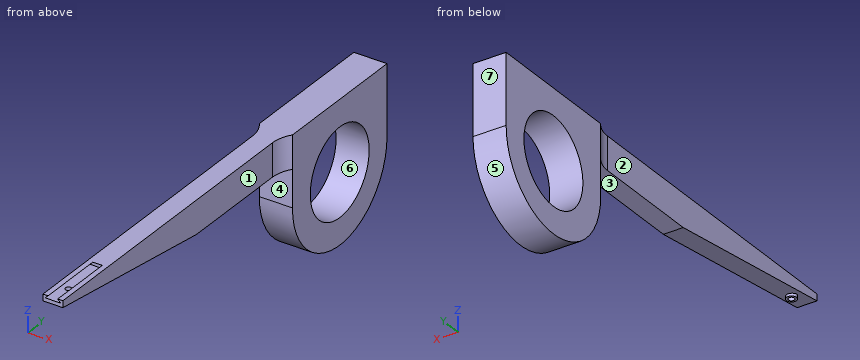
Autodesk Inventor part; units mm, degrees
ref_plane "YZ Plane" through (0, 0, 0) normal (1, 0, 0) x (0, 1, 0)
ref_plane "XZ Plane" through (0, 0, 0) normal (0, 1, 0) x (-1, 0, 0)
ref_plane "XY Plane" through (0, 0, 0) normal (0, 0, 1) x (1, 0, 0)
sketch "Sketch1" plane through (0, 0, 0) normal (1, 0, 0) x (0, 1, 0)
  circle A0 centre (0, 0) radius 6.604
  circle A1 centre (0, 0) radius 10.604
  line L0 (10.604, 0) -> (-10.604, 0)
  line L1 (-10.604, 0) -> (-10.604, 10.604)
  line L2 (-10.604, 10.604) -> (10.604, 10.604)
  line L3 (10.604, 10.604) -> (10.604, 0)
  point P0 (-10.604, 0)
  dimension "d1" = 21.208
  dimension "d0" = 13.208
extrude "Extrusion1" add sketch "Sketch1" along normal blind 5 contours L0 A1 A0 | A0 L0 A1 | A1 L2 L3 | L1 L2 A1
sketch "Sketch2" plane through (0, -10.604, 0) normal (0, -1, 0) x (1, 0, 0)
  line L0 (0, 0) -> (0, 10.604)
  line L1 (5, 0) -> (5, 10.604)
  line L2 (1, 10.604) -> (4, 10.604)
  line L3 (4, 10.604) -> (4, 5.604)
  line L4 (4, 5.604) -> (1, 5.604)
  line L5 (1, 5.604) -> (1, 10.604)
  line L6 (0, 10.604) -> (5, 10.604)
  dimension "d16" = 1
  dimension "d17" = 1
  dimension "d18" = 5
extrude "Extrusion2" add sketch "Sketch2" along normal blind 50
sketch "Sketch3" plane through (0, -60.604, 0) normal (0, -1, 0) x (1, 0, 0)
  line L0 (1.329, 10.154) -> (3.671, 10.154)
  line L1 (1.329, 10.154) -> (1.779, 10.604)
  line L2 (3.671, 10.154) -> (3.221, 10.604)
  line L3 (1.329, 10.154) -> (1.658, 10.154) construction
  line L4 (3.671, 10.154) -> (4, 10.154) construction
  line L5 (4, 10.604) -> (1, 10.604)
  line L6 (1.329, 10.154) -> (1, 10.154) construction
  line L7 (1, 10.604) -> (1, 5.604) construction
  line L8 (4, 5.604) -> (4, 10.604) construction
  point P0 (0, 0)
  dimension "d6" = 2.342
  dimension "d7" = 45
  dimension "d8" = 45
  dimension "d19" = 0.45
extrude "Extrusion3" cut sketch "Sketch3" against normal blind 10
chamfer "Chamfer1" distance 4 distance2 30 1 edges at (2.5, -60.604, 5.604) measured on face at (2.8903, -60.604, 7.1207)
fillet "Fillet1" radius 5 2 edges at (4, -10.604, 8.104) (1, -10.604, 8.104)
sketch "Sketch4" plane through (1.329, -60.604, 10.154) normal (0, 0, 1) x (1, 0, 0)
  circle A0 centre (1.171, 3.5) radius 0.45
  line L0 (1.171, 3.5) -> (2.671, 3.5) construction
  line L1 (1.171, 3.5) -> (-0.329, 3.5)
  line L2 (-0.329, 47) -> (-0.329, 0) construction
  line L3 (2.671, 47) -> (2.671, 0) construction
  line L4 (2.342, 0) -> (0, 0) construction
  point P0 (-1.329, 60.604)
  dimension "d21" = 0.9
  dimension "d22" = 3.5
extrude "Extrusion4" cut sketch "Sketch4" against normal blind 10
sketch "Sketch5" plane through (1.329, -60.604, 10.154) normal (0, 0, 1) x (1, 0, 0)
  circle A0 centre (1.171, 3.5) radius 0.45
  circle A1 centre (1.171, 3.5) radius 0.75
  point P0 (-1.329, 60.604)
  dimension "d25" = 1.5
extrude "Extrusion5" add sketch "Sketch5" against normal blind 1.5
equation "\"d17\" = d16"
equation "\"d8\" = d7"
properties part number "washing_arm"
Input: part model. Units: mm. Frame: model coordinates. Face numbers are marked on the shaded views. A direction names the side the tool comes from. Give positions to 0.01 mm unless a question says otherwise; leave off trailing zeros. Write each loop counter-clockwise with the first axis right and the second up, starting at its lowest first coordinate (ties: lowest second). Pieces come first, ordered by that corner, then holes. Notation, with made-up numbers: (77, 66.5) - (131, 66.5) arc R35 cw to (131, 103.5) - close; hole circle Ø3 at (74, 82.25). An arc over 180 degrees is marked (long way). Write item = value, one per line. Start each with the question number.
1) Cut plane C-C (y = -51.5). Return loops of the section in (x, z), and give its area (3 significant figures).
2) Reachability of the marked faces 1, 2 and 3 from +Z, -Z, +X, -X, +Y, -Y: full face, straight path, thin tool, end or side. Return the list, or none.
3) Cut plane D-D (y = -9.5). Return loops of the section in (x, z).
4) Pin query (flat end, axial travel): pin 1 (3 mm diameter, centred on x = 2, z = -3, fed in from -Y); pin 2 (12 mm diameter, centred on y = 0, z = 0, fed in from +X); pin 3 (1.6 mm diameter, centred on x = 2.5, y = -57, fed in from -Z); pin 4 (10 mm diameter, centred on y = -37, z = 8, fed in from +X). Return the tip coordinate at first contact, or that it passes through.
5) Material intervals for L1, parallel to Y at x = 2.5, z = 9.8; L2, parallel to Y at x = 3.75, z = 0; L3, parallel to Z at x = 1.8, y = -14.5, sorted ascending. Write a range as [from, to].
6) Cut plane B-B (y = -17). Return loops of the section in (x, z), and give its area (3 significant figures).
7) Cut plane A-A (y = 0). Return loops of the section in (x, z).
8) Draft query along Y for the marked faces 4, 5, 6 and 7. Return one class per face: pulls with the +Y half, pulls with the -Y half, needs draft (parallel to the pull), parting line crosses it, or undercut.
Answers follow:
q1.outline = (1, 8.39) - (4, 8.39) - (4, 10.6) - (3.22, 10.6) - (3.67, 10.15) - (1.33, 10.15) - (1.78, 10.6) - (1, 10.6) - close
q1.area = 5.79 mm^2
q2.face_1 = +Z, -Z, +X, -Y
q2.face_2 = +Z, -Z, -X, -Y
q2.face_3 = -Z, +X, -X, -Y
q3.outline = (0, -4.71) - (5, -4.71) - (5, 10.6) - (0, 10.6) - close
q4.pin_1 = -10.5
q4.pin_2 = through
q4.pin_3 = 8.65
q4.pin_4 = 4
q5.L1 = [-60.6, -57.55], [-56.65, 10.6]
q5.L2 = [-10.6, -6.6], [6.6, 10.6]
q5.L3 = [5.6, 10.6]
q6.outline = (1, 5.6) - (4, 5.6) - (4, 10.6) - (1, 10.6) - close
q6.area = 15.0 mm^2
q7.outline = (0, -10.6) - (5, -10.6) - (5, -6.6) - (0, -6.6) - close; (0, 6.6) - (5, 6.6) - (5, 10.6) - (0, 10.6) - close
q8.face_4 = pulls with the -Y half
q8.face_5 = parting line crosses it
q8.face_6 = undercut
q8.face_7 = pulls with the +Y half
